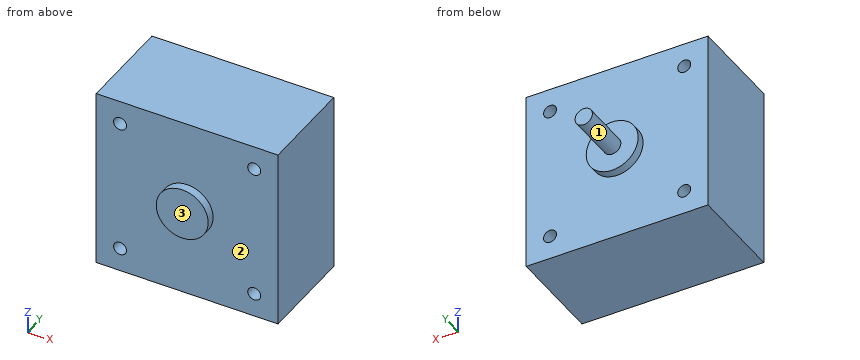
Autodesk Inventor part; units mm, degrees
ref_plane "YZ Plane" through (0, 0, 0) normal (1, 0, 0) x (0, 1, 0)
ref_plane "XZ Plane" through (0, 0, 0) normal (0, 1, 0) x (-1, 0, 0)
ref_plane "XY Plane" through (0, 0, 0) normal (0, 0, 1) x (1, 0, 0)
sketch "Sketch1" plane through (0, 0, 0) normal (0, 1, 0) x (-1, 0, 0)
  line L0 (0, 0) -> (42, 0)
  line L1 (42, 0) -> (42, -42)
  line L2 (42, -42) -> (0, -42)
  line L3 (0, -42) -> (0, 0)
  dimension "d0" = 42
  dimension "d1" = 42
extrude "Extrusion1" add sketch "Sketch1" along normal blind 22.5
sketch "Sketch2" plane through (0, 22.5, 0) normal (0, 1, 0) x (1, 0, 0)
  circle A0 centre (-21, 21) radius 6
  line L0 (-42, 42) -> (-42, 0)
  line L1 (-42, 0) -> (0, 0)
  point P0 (-42, 21)
  point P1 (-21, 0)
  dimension "d4" = 12
extrude "Extrusion2" add sketch "Sketch2" along normal blind 2 and the other way blind 24.5
sketch "Sketch3" plane through (-21, 24.5, -21) normal (0, 1, 0) x (1, 0, 0)
  circle A0 centre (0, 0) radius 2
  point P0 (21, -21)
  dimension "d7" = 4
extrude "Extrusion3" add sketch "Sketch3" along normal blind 11.5
sketch "Sketch4" plane through (0, 22.5, 0) normal (0, 1, 0) x (1, 0, 0)
  circle A0 centre (-5.5, 5.5) radius 1.5
  circle A1 centre (-36.5, 5.5) radius 1.5
  circle A2 centre (-36.5, 36.5) radius 1.5
  circle A3 centre (-5.5, 36.5) radius 1.5
  line L0 (0, 0) -> (0, 42)
  line L1 (0, 42) -> (-42, 42)
  line L2 (-42, 42) -> (-42, 0)
  line L3 (-42, 0) -> (0, 0)
  dimension "d10" = 3
  dimension "d11" = 3
  dimension "d12" = 3
  dimension "d13" = 3
  dimension "d14" = 31
  dimension "d15" = 31
  dimension "d16" = 5.5
  dimension "d17" = 5.5
  dimension "d22" = 31
  dimension "d23" = 31
  dimension "d24" = 5.5
  dimension "d25" = 5.5
  dimension "d26" = 5.5
  dimension "d27" = 5.5
extrude "Extrusion4" cut sketch "Sketch4" against normal up to next contours A0 | A1 | A2 | A3
properties part number "Motor"
Can you work these out from the model? Positions are in its coordinate system, mm. Face numbers are marked on the shaded views. A direction names the side the tool comes from. Give positions to 0.01 mm unless a question says otherwise; leave off trailing zeros. Write each loop counter-clockwise with the first axis right and the second up, starting at its lowest first coordinate (ties: lowest second). Pieces come first, ordered by that corner, then holes. Notation, with made-up numbers: (-27, -28.5) -> (-17, -28.5) arc R15 ccw to (-17, -17.5) -> close; hole circle Ø7 at (58, 81.25). An arc over 180 degrees is marked (long way). Answer as a JSON object with one key per item and string values. Group by question number.
Item 1: Suppose I cut it at D-D (x = -21). Please give me the cut outline in (y, z), plus the area to 3 significant figures.
Item 2: Suppose I cut it at C-C (y = 8). Please give me the cut outline in (x, z).
Item 3: Suppose I cut it at A-A (z = -36.5). Please give me the cut outline in (x, y).
Item 4: I'm going to push flat-ended pins straight in: P1, Ø1.5, axis at x = -22.5, z = -11, coming from the -Y side; P2, Ø8, axis at y = 27.5, z = -21, coming from the -X side; P3, Ø1.8, axis at x = -5.5, z = -5.5, coming from the -Y side; P4, Ø3.5, axis at x = -36.5, z = -36.5, coming from the +Y side. Where does each tip first touch, or does it pass through?
Item 5: Suppose I cut it at B-B (x = -36.5). Please give me the cut outline in (y, z).
Item 6: For the marked faces 1, 2 and 3, which set-ups out of +Z, -Z, +X, -X, +Y, -Y let a thin tool reach every point of the face, with its end or its side?
Item 7: Please list where these lines run through material, in increasing order: line 1 (Z direction, x = -36.5, y = 12); line 2 (Z direction, x = -36, y = 6). Write a range as [from, to].
Findings:
{
 "1": {"outline": "(-2, -27) -> (0, -27) -> (0, -42) -> (22.5, -42) -> (22.5, -27) -> (24.5, -27) -> (24.5, -23) -> (36, -23) -> (36, -19) -> (24.5, -19) -> (24.5, -15) -> (22.5, -15) -> (22.5, 0) -> (0, 0) -> (0, -15) -> (-2, -15) -> close", "area": "1,040 mm²"},
 "2": {"outline": "(-42, -42) -> (0, -42) -> (0, 0) -> (-42, 0) -> close; hole circle Ø3 at (-36.5, -36.5); hole circle Ø3 at (-36.5, -5.5); hole circle Ø3 at (-5.5, -36.5); hole circle Ø3 at (-5.5, -5.5)"},
 "3": {"outline": "(-42, 0) -> (-38, 0) -> (-38, 22.5) -> (-42, 22.5) -> close; (-35, 0) -> (-7, 0) -> (-7, 22.5) -> (-35, 22.5) -> close; (-4, 0) -> (0, 0) -> (0, 22.5) -> (-4, 22.5) -> close"},
 "4": {"P1": "stops at y = 0", "P2": "stops at x = -27", "P3": "passes through", "P4": "stops at y = 22.5"},
 "5": {"outline": "(0, -42) -> (22.5, -42) -> (22.5, -38) -> (0, -38) -> close; (0, -35) -> (22.5, -35) -> (22.5, -7) -> (0, -7) -> close; (0, -4) -> (22.5, -4) -> (22.5, 0) -> (0, 0) -> close"},
 "6": {"face 1": "+Y", "face 2": "-Y", "face 3": "+Z, -Z, +X, -X, -Y"},
 "7": {"line 1": "z = [-42, -38], [-35, -7], [-4, 0]", "line 2": "z = [-42, -37.91], [-35.09, -6.91], [-4.09, 0]"}
}
